```python
from build123d import *
from build123d.topology import SkipClean

# Parameters (mm, degrees)
ESQUISSE1_W             = 35
ESQUISSE1_H             = 39
BOSS_EXTRU_1_DEPTH      = 47
ENL_V_MAT_EXTRU_1_DEPTH = 20
CONG_1_R                = 17
ESQUISSE3_W             = 1
ESQUISSE3_H             = 20
ESQUISSE3_W_2           = 17
ENL_V_MAT_EXTRU_2_DEPTH = 7
ENL_V_MAT_EXTRU_3_DEPTH = 29
ESQUISSE5_R             = 4.5
ENL_V_MAT_EXTRU_4_DEPTH = 71.391760987
ESQUISSE7_R             = 11
ENL_V_MAT_EXTRU_5_DEPTH = 6
ENL_V_START             = -6
ESQUISSE8_R             = 11
ENL_V_MAT_EXTRU_6_DEPTH = 6
ENL_V_MAT_EXTRU_7_DEPTH = 6


with BuildPart() as part:
    # Esquisse1 → Boss.-Extru.1 (new body)
    with BuildSketch(Plane.XY):
        with Locations((17.5, -19.5)):
            Rectangle(ESQUISSE1_W, ESQUISSE1_H)
    extrude(amount=BOSS_EXTRU_1_DEPTH)

    # Esquisse2 → Enlèv. mat.-Extru.1 (cut)
    with BuildSketch(Plane.XY.offset(47)):
        with BuildLine():
            ThreePointArc((27.5, -19.5), (21.574863545, -10.367887041), (10.820902582, -12.057577163))
            Line((10.820902582, -12.057577163), (24.179097418, -26.942422837))
            ThreePointArc((24.179097418, -26.942422837), (26.632112959, -23.574863545), (27.5, -19.5))
        make_face()
        with BuildLine():
            Line((24.179097418, -26.942422837), (10.820902582, -12.057577163))
            ThreePointArc((10.820902582, -12.057577163), (10.057577163, -26.179097418), (24.179097418, -26.942422837))
        make_face()
    extrude(amount=-ENL_V_MAT_EXTRU_1_DEPTH, mode=Mode.SUBTRACT)

    # Congé1
    cong_1_edges = [part.edges().sort_by_distance(p)[0] for p in [
        (35, -19.5, 0),
        (0, -19.5, 0),
    ]]
    fillet(cong_1_edges, radius=CONG_1_R)

    # Esquisse3 → Enlèv. mat.-Extru.2 (cut)
    with BuildSketch(Plane(origin=(0, 0, 0), x_dir=(-1, 0, 0), z_dir=(0, 0, -1))):
        with Locations((-17.5, -19.5)):
            Rectangle(ESQUISSE3_W, ESQUISSE3_H)
        with Locations((-26.5, -19.5)):
            Rectangle(ESQUISSE3_W_2, ESQUISSE3_H)
        with Locations((-8.5, -19.5)):
            Rectangle(ESQUISSE3_W_2, ESQUISSE3_H)
    extrude(amount=-ENL_V_MAT_EXTRU_2_DEPTH, mode=Mode.SUBTRACT)

    # Esquisse4 → Enlèv. mat.-Extru.3 (cut)
    with BuildSketch(Plane(origin=(35, 0, 0), x_dir=(0, 0, -1), z_dir=(1, 0, 0))):
        with BuildLine():
            ThreePointArc((-18, -11), (-26.5, -19.5), (-18, -28))
            Line((-18, -28), (-18, -11))
        make_face()
        with BuildLine():
            Line((-17, -11.059028492), (-17, -27.940971508))
            ThreePointArc((-17, -27.940971508), (-11.645867486, -25.145794895), (-9.5, -19.5))
            ThreePointArc((-9.5, -19.5), (-11.645867486, -13.854205105), (-17, -11.059028492))
        make_face()
        with BuildLine():
            Line((-18, -11), (-18, -28))
            ThreePointArc((-18, -28), (-17.499129667, -27.985230045), (-17, -27.940971508))
            Line((-17, -27.940971508), (-17, -11.059028492))
            ThreePointArc((-17, -11.059028492), (-17.499129667, -11.014769955), (-18, -11))
        make_face()
    extrude(amount=-ENL_V_MAT_EXTRU_3_DEPTH, mode=Mode.SUBTRACT)

    # Esquisse5 → Enlèv. mat.-Extru.4 (cut, through all)
    with SkipClean():  # the faces are left unmerged after this step: merging them gives an invalid solid
        with BuildSketch(Plane(origin=(0, 0, 0), x_dir=(1, 0, 0), z_dir=(0, 1, 0))):
            with Locations(Location((17.5, -17.5, 0), (0, 0, 270))):
                Circle(ESQUISSE5_R)
        extrude(amount=-ENL_V_MAT_EXTRU_4_DEPTH, mode=Mode.SUBTRACT)

    # Esquisse7 → Enlèv. mat.-Extru.5 (cut)
    with SkipClean():  # the faces are left unmerged after this step: merging them gives an invalid solid
        with BuildSketch(Plane(origin=(0, 0, 0), x_dir=(1, 0, 0), z_dir=(0, 1, 0))):
            with Locations(Location((17.5, -17.5, 0), (0, 0, 270))):
                Circle(ESQUISSE7_R)
        extrude(amount=-ENL_V_MAT_EXTRU_5_DEPTH, mode=Mode.SUBTRACT)

    # Esquisse8 → Enlèv. mat.-Extru.6 (cut)
    with SkipClean():  # the faces are left unmerged after this step: merging them gives an invalid solid
        with BuildSketch(Plane.XZ.offset(39).offset(ENL_V_START)):
            with Locations(Location((17.5, 17.5, 0), (0, 0, 90))):
                Circle(ESQUISSE8_R)
        extrude(amount=ENL_V_MAT_EXTRU_6_DEPTH, mode=Mode.SUBTRACT)

    # Esquisse10 → Enlèv. mat.-Extru.7 (cut)
    with SkipClean():  # the faces are left unmerged after this step: merging them gives an invalid solid
        with BuildSketch(Plane.ZY):
            with BuildLine():
                ThreePointArc((17, -23.887482194), (20.80624304, -23.01781182), (22.5, -19.5))
                ThreePointArc((22.5, -19.5), (20.80624304, -15.98218818), (17, -15.112517806))
                Line((17, -15.112517806), (17, -23.887482194))
            make_face()
            with BuildLine():
                Line((17, -23.887482194), (17, -15.112517806))
                ThreePointArc((17, -15.112517806), (13.5, -19.5), (17, -23.887482194))
            make_face()
        extrude(amount=-ENL_V_MAT_EXTRU_7_DEPTH, mode=Mode.SUBTRACT)


solid = part.part
```
Work out the finished part from the listing and answer in its coordinate system (mm). A direction names the side the tool comes from. Round coordinates to 2 decimals unless told otherwise and drop trailing zeros. Loops run counter-clockwise (first coordinate to the right, second up) from the corner with the lowest first, then second, coordinate; pieces in that order, holes last. Notation, with made-up numbers: (-29, -23.75) -> (20, -23.75) arc R10 ccw to (20, -7.75) -> close; hole circle Ø5 at (-34, 15). An arc over 180 degrees is marked (long way). Write each question's results on one line, items separated by ' | '. Start each with the question number.
1. Find the intervals of material crossed by probe 1 along X at (y, z) = (-29.5, 17.5); probe 2 along Z at (x, y) = (17.5, -11); probe 3 along Y at (x, z) = (4, 17), in increasing order. Write a range as from..to.
2. Section B-B (x = 2) is taken. Determine the outline of the cut face in (y, z).
3. For a pull along Z with two mould halves and no side action, classify faces 1 (the face through (17, -9.5, 4)), 2 (the face through (2.97, -19.23, 7.4)), 3 (the face through (17.7, -6, 22.2)), 4 (the face through (27.259, -35.958, 22.576)) as +Z half, -Z half, draft (parallel to the pull), parting line (faces both ways), or undercut.
4. A tool of negligible diameter and unlimited length cuts with its end or side. For faces 5 (the face through (17.3, -33, 22.2)), 6 (the face through (7.741, -2.958, 22.576)), 7 (the face through (17, -19, 27)), from which of +Z, -Z, +X, -X, +Y, -Y can it reach the whole face along a straight path? Write none if from no direction.
5. Section C-C (z = 20.5) is taken. Determine the outline of the cut face in (x, y).
6. Section D-D (y = -18.5) is taken. Determine the outline of the cut face in (x, z), plus the area to 3 significant figures.
7. Given pin 1 Ø11 at (x, z) = (14, 15) entering from +Y; pin 2 Ø12 at (x, y) = (25, -29.5) entering from -Z; pin 3 Ø7 at (x, z) = (17.5, 17.5) entering from -Y; pin 4 Ø8 at (y, z) = (-14.5, 14.5) entering from +X, each flat-ended and moving along its own axis, determine where each tip first touches the part or whether it passes through.
8. Section A-A (y = -8.5) is taken. Determine the outline of the cut face in (x, z).
Evaluation:
1) probe 1: x = 0..13, 22..35 | probe 2: z = 7..13, 22..27 | probe 3: y = -39..-23.89, -15.11..0
2) outline: (-39, 9) -> (0, 9) -> (0, 47) -> (-39, 47) -> close; hole circle Ø9 at (-19.5, 18)
3) face 1: draft | face 2: -Z half | face 3: undercut | face 4: undercut
4) face 5: -Y | face 6: +Y | face 7: +Z
5) outline: (0, -39) -> (6.92, -39) -> (6.92, -33) -> (14.15, -33) -> (14.15, -27.62) -> (6, -27.62) -> (6, -23.24) -> (0, -23.24) -> close; (0, -15.76) -> (6, -15.76) -> (6, -11.38) -> (14.15, -11.38) -> (14.15, -6) -> (6.92, -6) -> (6.92, 0) -> (0, 0) -> close; (20.85, -33) -> (28.08, -33) -> (28.08, -39) -> (35, -39) -> (35, -27.62) -> (20.85, -27.62) -> close; (20.85, -11.38) -> (35, -11.38) -> (35, 0) -> (28.08, 0) -> (28.08, -6) -> (20.85, -6) -> close
6) outline: (0, 22.39) -> (6, 22.39) -> (6, 26.44) -> (35, 26.44) -> (35, 47) -> (27.45, 47) -> (27.45, 27) -> (7.55, 27) -> (7.55, 47) -> (0, 47) -> close; (0.34, 13.61) arc R17 ccw to (3.25, 7) -> (31.75, 7) arc R17 ccw to (33.29, 9.56) -> (6, 9.56) -> (6, 13.61) -> close | area: 444 mm2
7) pin 1: stops at y = -6 | pin 2: stops at z = 0.03 | pin 3: passes through | pin 4: stops at x = 35
8) outline: (0, 17) arc R17 ccw to (17, 0) -> (18, 0) arc R17 ccw to (35, 17) -> (35, 47) -> (0, 47) -> close; hole circle Ø9 at (17.5, 17.5)
